The figure shows three views and two pictorial views of one solid part (mm, origin at its lowest corner). Answer the questions. Coordinates: 2 decimals unless noted, no trailing zeros. Order: outer loops, then holes, each group sorted by start corner. A loop starts at its lowest first (then second) coordinate and runs counter-clockwise, first axis right, second up. Notation, with made-up numbers: M 24.5,43.5 L 53.5,43.5 A18 ccw 53.5,52.5 Z; hole C 79.25,57 d10. An arc over 180 degrees is marked long. Use a Markdown table: item, result.
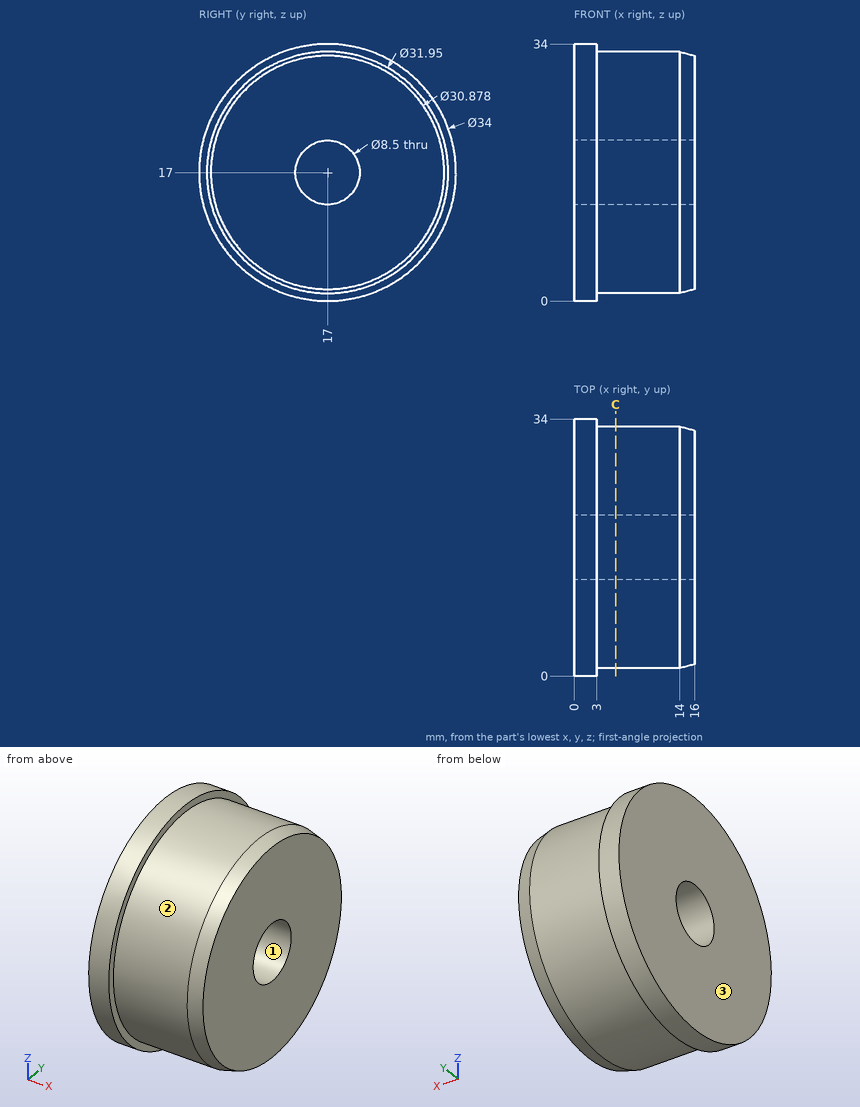
1. Find the intervals of material crossed by probe 1 along Z at (x, y) = (10.75, 17) (3 decimals); probe 2 along Z at (x, y) = (2.75, 18); probe 3 along X at (y, z) = (10.5, 32), in increasing order.
Answers below:
| item | result |
|---|---|
| probe 1 | 1.025 to 12.75, 21.25 to 32.975 |
| probe 2 | 0.03 to 12.87, 21.13 to 33.97 |
| probe 3 | 0 to 3 |
2. Section C-C on x = 5.5 is taken. Determine the outline of the cut face in (y, z) (3 decimals).
Answers below:
| item | result |
|---|---|
| outline | C 17,17 d31.95; hole C 17,17 d8.5 |
3. Flat-ended cylindrical pins translate along their axes: P1, Ø1.5, axis at x = 6, y = 6.5, coming from the +Z side (1 decimal); P2, Ø3, axis at x = 12, z = 3.5, coming from the +Y side (1 decimal); P3, Ø4, axis at x = 12.5, y = 28.5, coming from the +Z side. Find the tip coordinate at first contact, or state that the pin passes through.
Answers below:
| item | result |
|---|---|
| P1 | z = 29.7 |
| P2 | y = 27.5 |
| P3 | z = 29.84 |
4. For a pull along Y with two mould halves and no side action, classify the marked faces 1, 2 and 3 as +Y half, -Y half, draft (parallel to the pull), parting line (faces both ways), or undercut.
Answers below:
| item | result |
|---|---|
| face 1 | undercut |
| face 2 | parting line |
| face 3 | draft |
